Could you check a few things on this drawing? It's one solid part, dimensions in mm from its lowest x, y, z. Give positions to 0.01 mm unless a question says otherwise; leave off trailing zeros. Loops run counter-clockwise (first coordinate to the right, second up) from the corner with the lowest first, then second, coordinate; pieces in that order, holes last. Notation, with made-up numbers: (60, -37) - (119, -37) arc R23 ccw to (119, -28) - close; hole circle Ø9 at (-33, 59.5). An arc over 180 degrees is marked (long way). Write item = value, one per line.
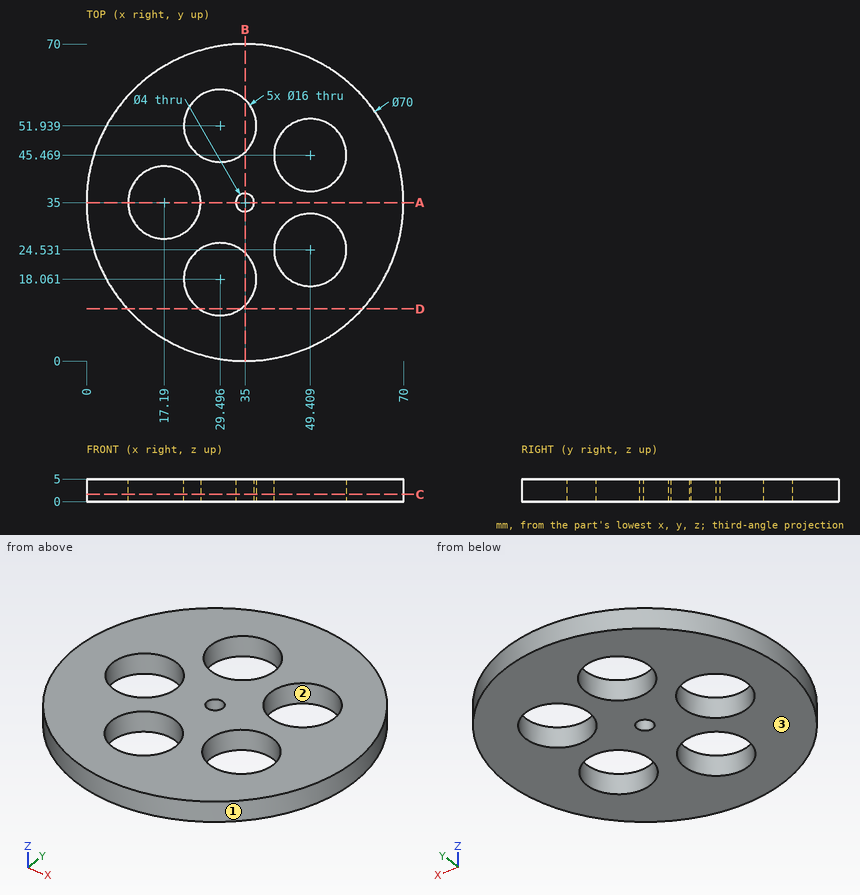
Q1. Imagine slicing it at B-B, the plane x = 35. Write out the boundary of the cut face in (y, z) (1 decimal), then the cut area to 3 significant figures.
Output:
outline = (0, 0) - (12.3, 0) - (12.3, 5) - (0, 5) - close; (23.9, 0) - (33, 0) - (33, 5) - (23.9, 5) - close; (37, 0) - (46.1, 0) - (46.1, 5) - (37, 5) - close; (57.7, 0) - (70, 0) - (70, 5) - (57.7, 5) - close
area = 214 mm2
Q2. For pin 1 (9.5 mm diameter, centred on x = 29.5, y = 18.06, fed in from -Z), with a flat end and sliding along its axis, tell me the tip position at first contact or that it passes through.
Output:
pin_1 = through
Q3. Imagine slicing it at C-C, the plane z = 1.6. Write out the boundary of the cut face in (x, y), then the cut area to 3 significant figures.
Output:
outline = circle Ø70 at (35, 35); hole circle Ø16 at (17.19, 35); hole circle Ø16 at (29.5, 18.06); hole circle Ø16 at (29.5, 51.94); hole circle Ø4 at (35, 35); hole circle Ø16 at (49.41, 24.53); hole circle Ø16 at (49.41, 45.47)
area = 2,830 mm2
Q4. We'd pull the mould along X, two halves only. Please class the marked faces 1, 2 and 3: released by +X, released by -X, zero draft, split by the parting line, or undercut.
Output:
face_1 = split by the parting line
face_2 = undercut
face_3 = zero draft
Q5. I need wall thicknesses on L1, parallel to X at y = 34.5, z = 3.15 (1 decimal); L2, parallel to Y at x = 56.5, z = 4.15 (1 decimal); L3, parallel to Y at x = 26, z = 3.25 (1 decimal). Which ranges of each line are inside material? Lowest first, please.
Output:
L1 = 0 to 9.2, 25.2 to 33.1, 36.9 to 70
L2 = 7.4 to 20.8, 28.2 to 41.8, 49.2 to 62.6
L3 = 1.2 to 10.9, 25.3 to 44.7, 59.1 to 68.8
Q6. Imagine slicing it at A-A, the plane y = 35. Write out the boundary of the cut face in (x, z).
Output:
outline = (0, 0) - (9.19, 0) - (9.19, 5) - (0, 5) - close; (25.19, 0) - (33, 0) - (33, 5) - (25.19, 5) - close; (37, 0) - (70, 0) - (70, 5) - (37, 5) - close
Q7. Imagine slicing it at D-D, the plane y = 11.5. Write out the boundary of the cut face in (x, z).
Output:
outline = (9.06, 0) - (24.92, 0) - (24.92, 5) - (9.06, 5) - close; (34.07, 0) - (60.94, 0) - (60.94, 5) - (34.07, 5) - close
